The model under review builds one solid part; all positions refer to its coordinate system, in mm. A direction names the side the tool comes from. Round coordinates to 2 decimals unless told otherwise and drop trailing zeros. Loops run counter-clockwise (first coordinate to the right, second up) from the corner with the lowest first, then second, coordinate; pieces in that order, holes last. Notation, with made-up numbers: (32.5, -0.75) -> (78.5, -0.75) arc R31 ccw to (78.5, 33.25) -> close; hole circle Ø9 at (77, 73.25). An arc over 180 degrees is marked (long way). Use a Markdown table: item, result. Add a question column.
1) Consider section B-B on y = 62.5. Give the boundary of the cut face in (x, z), plus the area to 3 significant figures.
2) Insertion check: pin 1 (4 mm diameter, centred on x = 394.5, y = 79.5, fed in from -Z); pin 2 (19.5 mm diameter, centred on x = 401, y = 131.5, fed in from +Z); pin 3 (10 mm diameter, centred on x = 331.5, z = 44, fed in from +Y). Each pin has a flat end and moves straight along its axis. Give the tip position at first contact, or say it passes through.
3) Consider section C-C on z = -47. Give the boundary of the cut face in (x, y).
4) Mouldability with a two-part tool opening along Y and no side actions: class faces 1 (the flat face through (419.05, 12.053, -41.785)), 2 (the flat face through (419, 67, 16.883)), 3 (the flat face through (419, 134, -38.704)), 4 (the flat face through (419, 145.71, 0)) as released by +Y, released by -Y, zero draft, split by the parting line, or undercut.
5) Consider section A-A on x = 590.5. Give the boundary of the cut face in (y, z), plus the area to 3 significant figures.
6) For faces 5 (the flat face through (419.05, 122.058, -27.641)), 6 (the flat face through (419.05, 122.145, 27.947)), 7 (the flat face through (850, 74, 1)), 8 (the flat face through (0, 74, 1)), 9 (the flat face through (419, 134, 38.704)), list the 3-axis set-ups (+Z, -Z, +X, -X, +Y, -Y) from which the entire face can be reached by the end or side of a thin tool; tool diameter is ignored.
7) Wall thickness on probe 1 along Z at (x, y) = (690, 126); probe 2 along Z at (x, y) = (327.5, 81.5); probe 3 along Y at (x, z) = (512, -37.5): over which ranges is each line inside the solid? List them lowest first.
from build123d import *

# Parameters (mm, degrees)
EXTRUDE_1_DEPTH = 850


with BuildPart() as part:
    # Эскиз1 → Бобышка-Вытянуть1 (new body)
    with BuildSketch(Plane(origin=(0, 0, 0), x_dir=(0, 0, -1), z_dir=(1, 0, 0))):
        Polygon((-66, 0), (66, 0), (66, 10), (16.883336969, 14.163502235), (16.883336969, 118.984443331), (38.704461372, 125.219050303), (38.704461372, 142.782419329), (34.150995328, 145.7096475), (-34.150995328, 145.7096475), (-38.704461372, 142.782419329), (-38.704461372, 125.219050303), (-16.883336969, 118.984443331), (-16.883336969, 14.163502235), (-66, 10), align=None)
    extrude(amount=EXTRUDE_1_DEPTH)


solid = part.part
Result set:
| question | item | result |
|---|---|---|
| 1 | outline | (0, -16.88) -> (850, -16.88) -> (850, 16.88) -> (0, 16.88) -> close |
| 1 | area | 28,700 mm2 |
| 2 | pin 1 | z = -16.88 |
| 2 | pin 2 | z = 38.7 |
| 2 | pin 3 | y = 12.29 |
| 3 | outline | (0, 0) -> (850, 0) -> (850, 11.61) -> (0, 11.61) -> close |
| 4 | face 1 | undercut |
| 4 | face 2 | undercut |
| 4 | face 3 | zero draft |
| 4 | face 4 | released by +Y |
| 5 | outline | (0, -66) -> (10, -66) -> (14.16, -16.88) -> (118.98, -16.88) -> (125.22, -38.7) -> (142.78, -38.7) -> (145.71, -34.15) -> (145.71, 34.15) -> (142.78, 38.7) -> (125.22, 38.7) -> (118.98, 16.88) -> (14.16, 16.88) -> (10, 66) -> (0, 66) -> close |
| 5 | area | 7,120 mm2 |
| 6 | face 5 | -Z, +X, -X |
| 6 | face 6 | +Z, +X, -X |
| 6 | face 7 | +Z, -Z, +X, +Y, -Y |
| 6 | face 8 | +Z, -Z, -X, +Y, -Y |
| 6 | face 9 | +Z, +X, -X, +Y |
| 7 | probe 1 | -38.7 to 38.7 |
| 7 | probe 2 | -16.88 to 16.88 |
| 7 | probe 3 | 0 to 12.42, 124.87 to 143.56 |
